Could you check a few things on this model? Use its own coordinates, in mm. Give positions to 0.01 mm unless a question says otherwise; leave off trailing zeros. Write item = value, one per line.
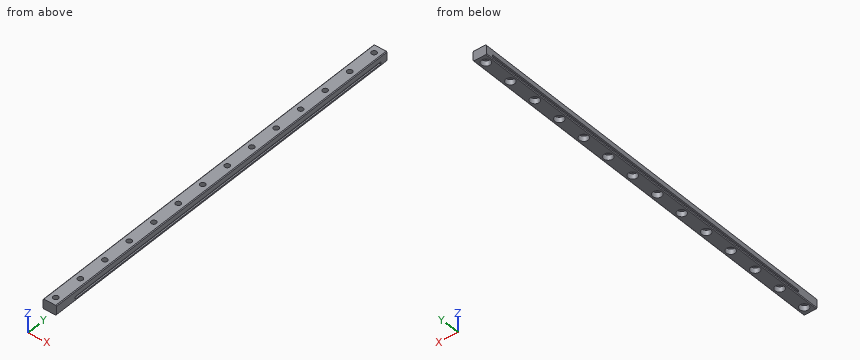
from build123d import *

# Parameters (mm, degrees)
EXTRUDE_1_DEPTH          = 130
EXTRUDE_1_DEPTH_BACK     = 140
SKETCH_1_W               = 9
SKETCH_1_H               = 6.5
CUT_EXTRUDE_1_DEPTH      = 125
CUT_EXTRUDE_1_DEPTH_BACK = 125
SKETCH_2_W               = 0.95
SKETCH_2_H               = 1.48
CHAMFER_2_SIZE           = 0.5
SKETCH_3_R               = 3
CUT_EXTRUDE_2_DEPTH      = 3.5
SKETCH_4_R               = 1.75
CUT_EXTRUDE_3_DEPTH      = 5


with BuildPart() as part:
    # 草图1 → 凸台-拉伸1 (new, two sides: drawn at the far end of the back side and taken through both)
    with BuildSketch(Plane(origin=(0, 0, 0), x_dir=(1, 0, 0), z_dir=(0, 1, 0)).offset(-EXTRUDE_1_DEPTH_BACK)):
        Rectangle(SKETCH_1_W, SKETCH_1_H)
    extrude(amount=EXTRUDE_1_DEPTH + EXTRUDE_1_DEPTH_BACK)

    # 草图2 → 切除-拉伸1 (cut, two sides: drawn at the far end of the back side and taken through both)
    with BuildSketch(Plane(origin=(0, 0, 0), x_dir=(1, 0, 0), z_dir=(0, 1, 0)).offset(-CUT_EXTRUDE_1_DEPTH_BACK)):
        with Locations((4.025, 1.15)):
            Rectangle(SKETCH_2_W, SKETCH_2_H)
        with Locations((-4.025, 1.15)):
            Rectangle(SKETCH_2_W, SKETCH_2_H)
    extrude(amount=CUT_EXTRUDE_1_DEPTH + CUT_EXTRUDE_1_DEPTH_BACK, mode=Mode.SUBTRACT)

    # 倒角2
    chamfer_2_edges = [part.edges().sort_by_distance(p)[0] for p in [
        (4.5, -5, 3.25),
        (-4.5, -5, 3.25),
        (-4.5, -5, -3.25),
        (4.5, -5, -3.25),
    ]]
    chamfer(chamfer_2_edges, length=CHAMFER_2_SIZE)

    # 草图3 → 切除-拉伸2 (cut)
    with BuildSketch(Plane(origin=(0, 0, -3.25), x_dir=(-1, 0, 0), z_dir=(0, 0, -1))):
        with Locations((0, -135)):
            Circle(SKETCH_3_R)
        with Locations((0, -115)):
            Circle(SKETCH_3_R)
        with Locations((0, -95)):
            Circle(SKETCH_3_R)
        with Locations((0, -75)):
            Circle(SKETCH_3_R)
        with Locations((0, -55)):
            Circle(SKETCH_3_R)
        with Locations((0, -35)):
            Circle(SKETCH_3_R)
        with Locations((0, -15)):
            Circle(SKETCH_3_R)
        with Locations((0, 5)):
            Circle(SKETCH_3_R)
        with Locations((0, 25)):
            Circle(SKETCH_3_R)
        with Locations((0, 45)):
            Circle(SKETCH_3_R)
        with Locations((0, 65)):
            Circle(SKETCH_3_R)
        with Locations((0, 85)):
            Circle(SKETCH_3_R)
        with Locations((0, 105)):
            Circle(SKETCH_3_R)
        with Locations((0, 125)):
            Circle(SKETCH_3_R)
    extrude(amount=-CUT_EXTRUDE_2_DEPTH, mode=Mode.SUBTRACT)

    # 草图4 → 切除-拉伸3 (cut)
    with BuildSketch(Plane(origin=(0, 0, 0.25), x_dir=(-1, 0, 0), z_dir=(0, 0, -1))):
        with Locations((0, -135)):
            Circle(SKETCH_4_R)
        with Locations((0, -115)):
            Circle(SKETCH_4_R)
        with Locations((0, -95)):
            Circle(SKETCH_4_R)
        with Locations((0, -75)):
            Circle(SKETCH_4_R)
        with Locations((0, -55)):
            Circle(SKETCH_4_R)
        with Locations((0, -35)):
            Circle(SKETCH_4_R)
        with Locations((0, -15)):
            Circle(SKETCH_4_R)
        with Locations((0, 5)):
            Circle(SKETCH_4_R)
        with Locations((0, 25)):
            Circle(SKETCH_4_R)
        with Locations((0, 45)):
            Circle(SKETCH_4_R)
        with Locations((0, 65)):
            Circle(SKETCH_4_R)
        with Locations((0, 85)):
            Circle(SKETCH_4_R)
        with Locations((0, 105)):
            Circle(SKETCH_4_R)
        with Locations((0, 125)):
            Circle(SKETCH_4_R)
        with Locations((0, 145)):
            Circle(SKETCH_4_R)
    extrude(amount=-CUT_EXTRUDE_3_DEPTH, mode=Mode.SUBTRACT)


solid = part.part
1. If we section it at A-A, the plane x = 0: Count the separate pieces of the cut face and the enclosed holes in it, and give its area (3 significant figures).
Filled sheet:
separate_pieces = 15
enclosed_holes = 0
area = 1,310 mm2
2. I need wall thicknesses on line 1 (Z direction, x = -3.75, y = -92.5); line 2 (X direction, y = -135, z = -1.2); line 3 (X direction, y = -39, z = -0.75). Which ranges of each line are inside material? Lowest first, please.
Filled sheet:
line_1 = -3.25 to -1.89, -0.41 to 3.25
line_2 = -4.5 to -3, 3 to 4.5
line_3 = -3.55 to 3.55
3. For pin 1 (3 mm diameter, centred on x = 0.5, y = -74.5, fed in from -Z); pin 2 (2 mm diameter, centred on x = 0, y = -75, fed in from -Z) (3 decimals), each with a flat end and sliding along its axis, tell me the tip position at first contact or that it passes through.
Filled sheet:
pin_1 = 0.25
pin_2 = through
